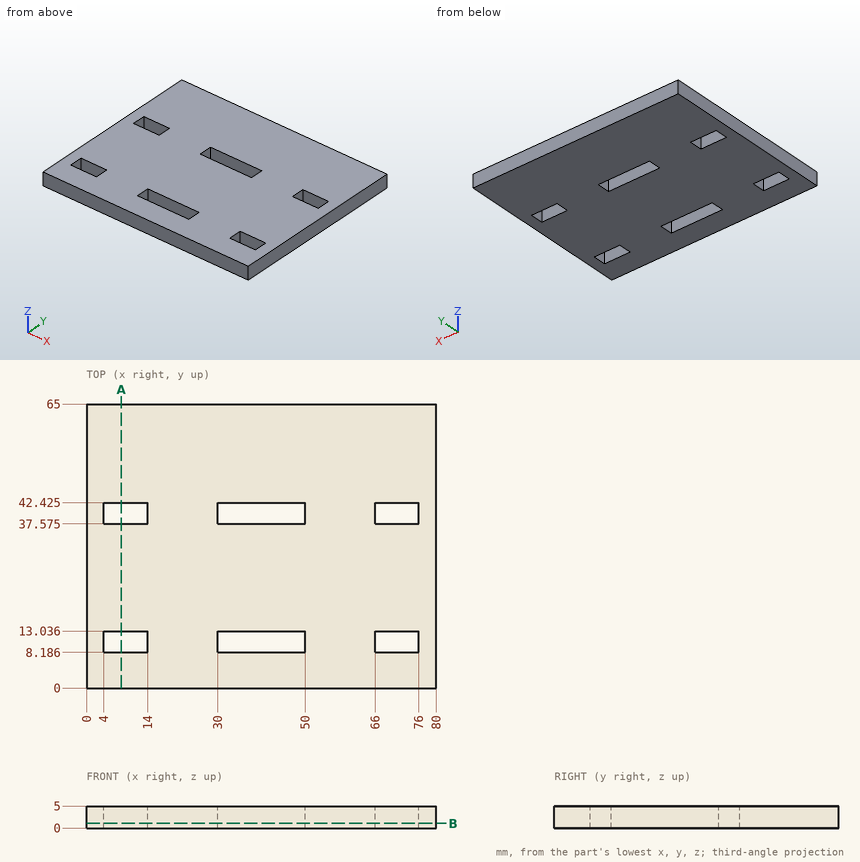
Geometry: see drawing. Coordinates: mm, zero at the bounding-box minimum. Round coordinates to 2 decimals unless told otherwise and drop trailing zeros. Write each loop counter-clockwise with the first axis right and the second up, starting at its lowest first coordinate (ties: lowest second). Pieces come first, ordered by that corner, then holes. Notation, with made-up numbers: (89.5, -15.75) - (115.5, -15.75) arc R30 ccw to (115.5, 19.25) - close; hole circle Ø3 at (60, 87). An arc over 180 degrees is marked (long way). Use CSV: the item, a comma, the result in double quotes. Start each with the question number.
(1) First-contact query: pin 1 Ø1.5 at (x, y) = (10.5, 11.5) entering from -Z. Flat tip, straight axial feed; report the tip coordinate or a pass-through.
(2) Cut plane B-B, the plane z = 1.1. Return loops of the section in (x, y) (3 decimals).
(3) Cut plane A-A, the plane x = 8. Return loops of the section in (y, z) (3 decimals), and give its area (4 significant figures).
(4) Material intervals for probe 1 along Y at (x, z) = (46.5, 3.2) (3 decimals); probe 2 along X at (y, z) = (11.5, 2), sorted ascending. Write a range as [from, to].
Geometry says:
1,pin 1,"through"
2,outline,"(0, 0) - (80, 0) - (80, 65) - (0, 65) - close; hole (4, 8.186) - (14, 8.186) - (14, 13.036) - (4, 13.036) - close; hole (4, 37.575) - (14, 37.575) - (14, 42.425) - (4, 42.425) - close; hole (30, 8.186) - (50, 8.186) - (50, 13.036) - (30, 13.036) - close; hole (30, 37.575) - (50, 37.575) - (50, 42.425) - (30, 42.425) - close; hole (66, 8.186) - (76, 8.186) - (76, 13.036) - (66, 13.036) - close; hole (66, 37.575) - (76, 37.575) - (76, 42.425) - (66, 42.425) - close"
3,outline,"(0, 0) - (8.186, 0) - (8.186, 5) - (0, 5) - close; (13.036, 0) - (37.575, 0) - (37.575, 5) - (13.036, 5) - close; (42.425, 0) - (65, 0) - (65, 5) - (42.425, 5) - close"
3,area,"276.5 mm²"
4,probe 1,"[0, 8.186], [13.036, 37.575], [42.425, 65]"
4,probe 2,"[0, 4], [14, 30], [50, 66], [76, 80]"
